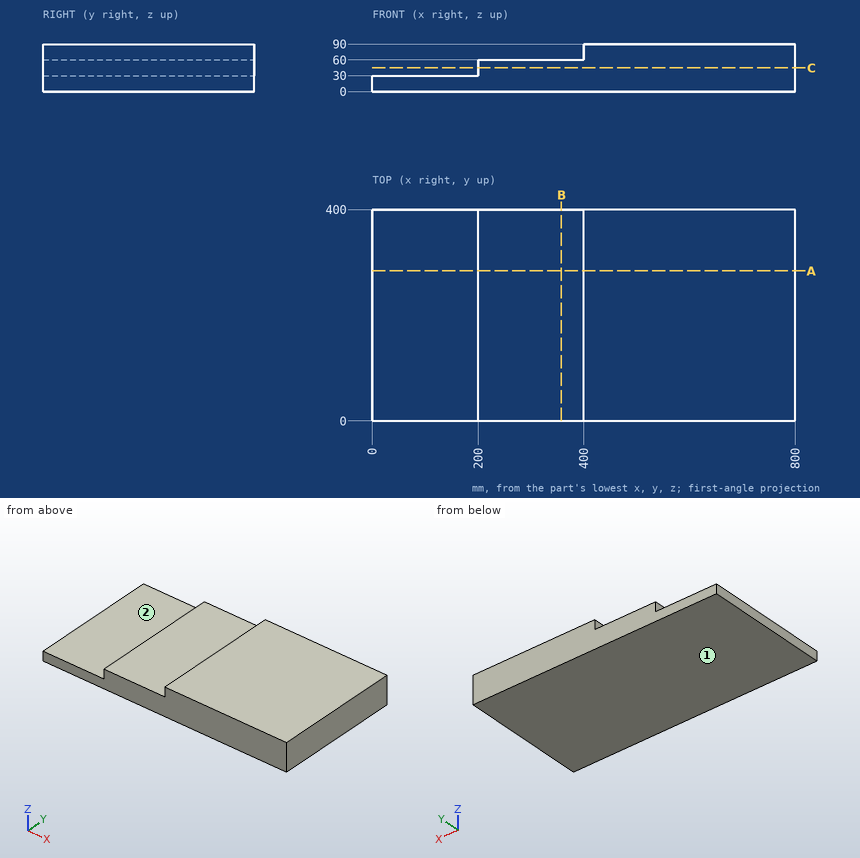
The drawing under review shows one solid part. Ordinate dimensions are in mm from its lowest x, y, z. A direction names the side the tool comes from. Coordinates: 2 decimals unless noted, no trailing zeros. Order: outer loops, then holes, each group sorted by start corner. A loop starts at its lowest first (then second) coordinate and runs counter-clockwise, first axis right, second up. Notation, with made-up numbers: (28, 13.5) -> (87, 13.5) arc R24 ccw to (87, 48.5) -> close; hole circle Ø8 at (-25.75, 89). An arc over 180 degrees is marked (long way). Use CSV: the item, a comma, the result in double quotes. Start each with the question number.
Item 1: We need section B-B, the plane x = 358. Give the boundary of the cut face in (y, z), then the cut area to 3 significant figures.
Item 2: For the marked faces 1 and 2, list the 3-axis set-ups (+Z, -Z, +X, -X, +Y, -Y) from which the entire face can be reached by the end or side of a thin tool; tool diameter is ignored.
Item 3: Wall thickness on probe 1 along X at (y, z) = (221, 86.5); probe 2 along Z at (x, y) = (56, 272); probe 3 along X at (y, z) = (338, 32): over which ranges is each line inside the solid? List them lowest first.
Item 4: We need section C-C, the plane z = 45. Give the boundary of the cut face in (x, y).
Item 5: Insertion check: pin 1 (9 mm diameter, centred on y = 249.5, z = 82, fed in from -X); pin 2 (5 mm diameter, centred on y = 63, z = 44.5, fed in from -X). Each pin has a flat end and moves straight along its axis. Give the tip position at first contact, or say it passes through.
Item 6: We need section A-A, the plane y = 284. Give the boundary of the cut face in (x, z).
Derived:
1,outline,"(0, 0) -> (400, 0) -> (400, 60) -> (0, 60) -> close"
1,area,"24,000 mm^2"
2,face 1,"-Z, +X, -X, +Y, -Y"
2,face 2,"+Z, -X, +Y, -Y"
3,probe 1,"x = 400 to 800"
3,probe 2,"z = 0 to 30"
3,probe 3,"x = 200 to 800"
4,outline,"(200, 0) -> (800, 0) -> (800, 400) -> (200, 400) -> close"
5,pin 1,"stops at x = 400"
5,pin 2,"stops at x = 200"
6,outline,"(0, 0) -> (800, 0) -> (800, 90) -> (400, 90) -> (400, 60) -> (200, 60) -> (200, 30) -> (0, 30) -> close"
